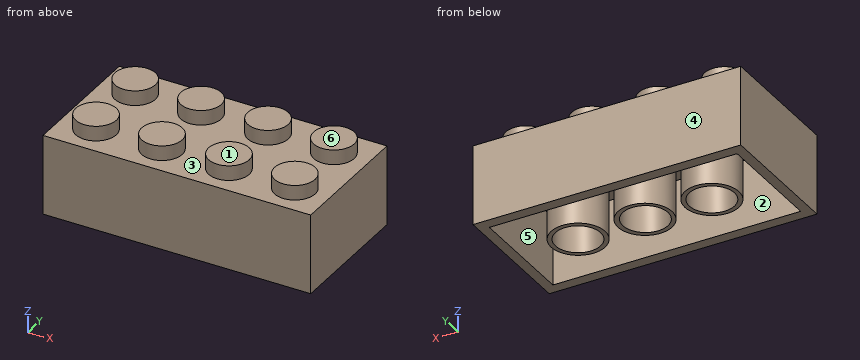
```python
from build123d import *

# Parameters (mm, degrees)
F0_W     = 31.6738
F0_H     = 15.748
F1_DEPTH = 9.4488
F2_R     = 2.4003
F3_DEPTH = 1.7526
F4_W     = 29.3116
F4_H     = 13.1318
F5_DEPTH = 8.128
F6_R     = 3.1877
F7_DEPTH = 8.128
F8_R     = 2.667
F9_DEPTH = 8.128


with BuildPart() as f1:
    # F0 (on Top) → F1 (new body)
    with BuildSketch(Plane.XY):
        Rectangle(F0_W, F0_H)
    extrude(amount=F1_DEPTH)

    # F2 (on face) → F3 (join)
    with BuildSketch(Plane.XY.offset(9.4488)):
        with Locations((-11.7602, 4.036113)):
            Circle(F2_R)
        with Locations((3.9624, -4.036113)):
            Circle(F2_R)
        with Locations((3.9624, 4.036113)):
            Circle(F2_R)
        with Locations((-3.9624, 4.036113)):
            Circle(F2_R)
        with Locations((-3.9624, -4.036113)):
            Circle(F2_R)
        with Locations((-11.7602, -4.036113)):
            Circle(F2_R)
        with Locations((11.7602, -4.036113)):
            Circle(F2_R)
        with Locations((11.7602, 4.036113)):
            Circle(F2_R)
    extrude(amount=F3_DEPTH)

    # F4 (on face) → F5 (cut)
    with BuildSketch(Plane(origin=(0, 0, 0), x_dir=(1, 0, 0), z_dir=(0, 0, -1))):
        Rectangle(F4_W, F4_H)
    extrude(amount=-F5_DEPTH, mode=Mode.SUBTRACT)

    # F6 (on face) → F7 (join)
    with BuildSketch(Plane(origin=(0, 0, 8.128), x_dir=(1, 0, 0), z_dir=(0, 0, -1))):
        with Locations((-7.9121, 0)):
            Circle(F6_R)
        with Locations((7.9121, 0)):
            Circle(F6_R)
        Circle(F6_R)
    extrude(amount=F7_DEPTH)

    # F8 (on face) → F9 (cut)
    with BuildSketch(Plane(origin=(0, 0, 0), x_dir=(1, 0, 0), z_dir=(0, 0, -1))):
        with Locations((-7.9121, 0)):
            Circle(F8_R)
        with Locations((-0.064154, -0.027935)):
            Circle(F8_R)
        with Locations((7.9257, 0)):
            Circle(F8_R)
    extrude(amount=-F9_DEPTH, mode=Mode.SUBTRACT)


solid = f1.part
```
The listing builds one solid part. Answer for the finished solid, in the listing's coordinates (mm). Face numbers are marked on the shaded views. A direction names the side the tool comes from. Give positions to 0.01 mm unless a question says otherwise; leave off trailing zeros. Order: outer loops, then holes, each group sorted by start corner. A loop starts at its lowest first (then second) coordinate and runs counter-clockwise, first axis right, second up. Notation, with made-up numbers: (-14.5, 36) -> (15.5, 36) arc R26 ccw to (15.5, 51) -> close; hole circle Ø11 at (32.25, -20.75). An arc over 180 degrees is marked (long way). Answer as a JSON object with one key per item and string values. Group by question number.
Item 1: A tool of negligible diameter and unlimited length cuts with its end or side. For the marked faces 5 and 6, from which of +Z, -Z, +X, -X, +Y, -Y can it reach the whole face along a straight path? Write none if from no direction.
Item 2: The part is cut by section D-D on x = 8.5. Write down the section's boundary in (y, z).
Item 3: Consider L1, parallel to Y at x = -1.5, z = 2.25; L2, parallel to Y at x = -7, z = 2.5; L3, parallel to X at y = -3.75, z = 10. Determine where each line is inside the solid, lowest interval first. Write a range as from..to.
Item 4: A flat-ended cylindrical pin translates along its axis: pin 1 (1.6 mm diameter, centred on x = -9, y = -1, fed in from -Z). Find the tip coordinate at first contact, or state that the pin passes through.
Item 5: The part is cut by section A-A on z = 6. Write down the section's boundary in (x, y).
Item 6: Determine the mould class of the marked faces 1, 2, 3 and 4 for opening direction Y: pulls with the +Y half, pulls with the -Y half, needs draft (parallel to the pull), parting line crosses it, or undercut.
Item 7: The part is cut by section C-C on x = 12.5. Write down the section's boundary in (y, z).
Result set:
{
 "1": {"face 5": "-Z", "face 6": "+Z, +X, -X, +Y, -Y"},
 "2": {"outline": "(-7.87, 0) -> (-6.57, 0) -> (-6.57, 8.13) -> (-3.13, 8.13) -> (-3.13, 0) -> (-2.6, 0) -> (-2.6, 8.13) -> (2.6, 8.13) -> (2.6, 0) -> (3.13, 0) -> (3.13, 8.13) -> (6.57, 8.13) -> (6.57, 0) -> (7.87, 0) -> (7.87, 9.45) -> (-7.87, 9.45) -> close"},
 "3": {"L1": "-7.87..-6.57, -2.81..-2.22, 2.28..2.81, 6.57..7.87", "L2": "-7.87..-6.57, -3.05..-2.51, 2.51..3.05, 6.57..7.87", "L3": "-14.14..-9.38, -6.35..-1.58, 1.58..6.35, 9.38..14.14"},
 "4": {"pin 1": "z = 8.13"},
 "5": {"outline": "(-15.84, -7.87) -> (15.84, -7.87) -> (15.84, 7.87) -> (-15.84, 7.87) -> close; circle Ø6.38 at (-7.91, 0); circle Ø6.38 at (0, 0); circle Ø6.38 at (7.91, 0); hole (-14.66, -6.57) -> (14.66, -6.57) -> (14.66, 6.57) -> (-14.66, 6.57) -> close; hole circle Ø5.33 at (-7.91, 0); hole circle Ø5.33 at (-0.06, 0.03); hole circle Ø5.33 at (7.93, 0)"},
 "6": {"face 1": "needs draft", "face 2": "undercut", "face 3": "undercut", "face 4": "pulls with the +Y half"},
 "7": {"outline": "(-7.87, 0) -> (-6.57, 0) -> (-6.57, 8.13) -> (6.57, 8.13) -> (6.57, 0) -> (7.87, 0) -> (7.87, 9.45) -> (6.32, 9.45) -> (6.32, 11.2) -> (1.75, 11.2) -> (1.75, 9.45) -> (-1.75, 9.45) -> (-1.75, 11.2) -> (-6.32, 11.2) -> (-6.32, 9.45) -> (-7.87, 9.45) -> close"}
}
